Autodesk Inventor part; units mm, degrees
ref_plane "YZ Plane" through (0, 0, 0) normal (1, 0, 0) x (0, 1, 0)
ref_plane "XZ Plane" through (0, 0, 0) normal (0, 1, 0) x (-1, 0, 0)
ref_plane "XY Plane" through (0, 0, 0) normal (0, 0, 1) x (1, 0, 0)
sketch "Schizzo1" plane through (0, 0, 0) normal (0, 0, 1) x (1, 0, 0)
  circle A0 centre (0, 0) radius 9
  dimension "diametro" = 18
extrude "Estrusione1" add sketch "Schizzo1" along normal mid plane 74
sketch "Schizzo2" plane through (0, 0, 0) normal (1, 0, 0) x (0, 1, 0)
  line L0 (0, 0) -> (0, -36.2228) construction
  line L1 (0, 0) -> (14.2779, 0) construction
  point P0 (0, -31)
  point P1 (0, 31)
  dimension "L1" = 62
hole "Foro1" at (0, 0, -31) at (0, 0, 31) direction (-1, 0, 0) diameter 6 end through all both
chamfer "Smusso1" distance 0.5 angle 45 8 edges at (-9, 0, 37) (-9, 0, -37) (8.4853, -3, 31) (8.4853, 3, 31) (-9, 0.0004, 34) (8.4853, 3, -31) (8.4853, -3, -31) (-9, 0.0004, -28)
properties part number "05-16-2023 Perno-02"
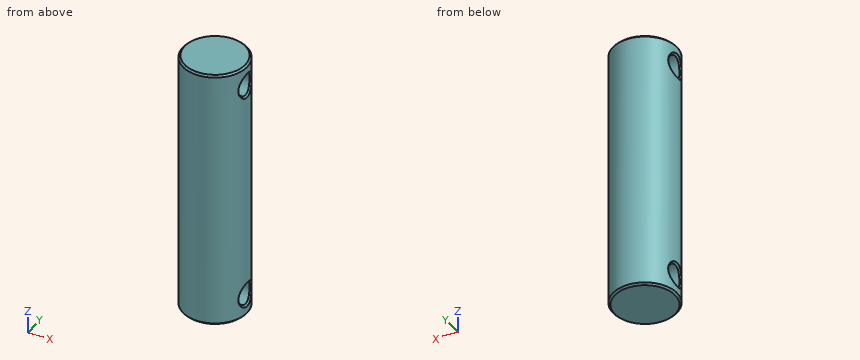
Model file for the job. Use its own axes, mm. Round coordinates to 2 decimals unless told otherwise and drop trailing zeros. Order: outer loops, then holes, each group sorted by start corner. A loop starts at its lowest first (then second) coordinate and runs counter-clockwise, first axis right, second up. Notation, with made-up numbers: M 83.5,65.25 L 95.5,65.25 A16 cw 95.5,95.25 Z; hole C -6.5,11 d7. An arc over 180 degrees is marked long. Write each question's results on one line, items separated by ' | '. Start each with the question number.
(1) Saw through at A-A, the plane x = 0. Give the cut face in (y, z), then the cut area to 3 significant figures.
(2) Drop flat-ended pins along their axis: pin 1 (5 mm diameter, centred on y = 0, z = -31, fed in from -X); pin 2 (1 mm diameter, centred on x = 6, z = -17.5, fed in from -Y); pin 3 (8 mm diameter, centred on x = -7, z = 8, fed in from +Y); pin 4 (2 mm diameter, centred on y = -7, z = 8, fed in from -X). Give the stop position or say it passes through.
(3) Saw through at C-C, the plane y = 2. State how many separate pieces and enclosed holes the cut face has, then the cut area to 3 significant figures.
(4) Saw through at B-B, the plane z = -1.5. Give the cut face in (x, y).
(5) Probe probe 1 along Z at (x, y) = (3.5, 0); probe 2 along Y at (x, z) = (0.5, 31); probe 3 along Z at (x, y) = (-5.75, 0.75). List the from-to ranges inside material, lowest first. Write a range as from..to.
Established:
1) outline: M -9,-36.5 L -8.5,-37 L 8.5,-37 L 9,-36.5 L 9,36.5 L 8.5,37 L -8.5,37 L -9,36.5 Z; hole C 0,-31 d6; hole C 0,31 d6 | area: 1,270 mm^2
2) pin 1: passes through | pin 2: stops at y = -7.12 | pin 3: stops at y = 8.49 | pin 4: stops at x = -6.71
3) separate pieces: 3 | enclosed holes: 0 | area: 1,140 mm^2
4) outline: C 0,0 d18
5) probe 1: z = -37..-34, -28..28, 34..37 | probe 2: y = -8.99..-3, 3..8.99 | probe 3: z = -37..-33.9, -28.1..28.1, 33.9..37
